Could you check a few things on this model? Use its own coordinates, in mm. Face numbers are marked on the shaded views. A direction names the side the tool comes from. Give positions to 0.01 mm unless a question says otherwise; leave off trailing zeros. Order: outer loops, then holes, each group sorted by start corner. A loop starts at its lowest first (then second) coordinate and runs counter-clockwise, first axis right, second up.
(1) If I drill on probe 1 along Z at (x, y) = (9, 15), over which ranges is the centre line in solid material (lowest first)?
(2) On a 3-axis mill with a long thin cutter (end or side, diameter ignored), from which of +Z, -Z, +X, -X, +Y, -Y can I reach the whole of each face in a straight line? I mean the marked faces 4 and 5. Say none if no direction works.
(3) Imagine slicing it at A-A, the plane x = 2. Write out the boundary of the cut face in (y, z).
(4) Will these pins go through, and if not, where does the flat tip stop? pin 1 (6 mm diameter, centred on y = 11.5, z = 2, fed in from -X); pin 2 (6 mm diameter, centred on x = 8.5, y = 12, fed in from +Z).
(5) Imagine slicing it at D-D, the plane x = 15.5. Write out the boundary of the cut face in (y, z).
(6) If we mould it in two halves opening along Y, with no side actions, what happens to the marked faces 1, 2 and 3? For each: released by +Y, released by -Y, zero draft, split by the parting line, or undercut.
(7) Imagine slicing it at B-B, the plane y = 2. Write out the boundary of the cut face in (x, z), then the cut area to 3 significant figures.
(8) Imagine slicing it at C-C, the plane y = 17.75. Write out the boundary of the cut face in (x, z).
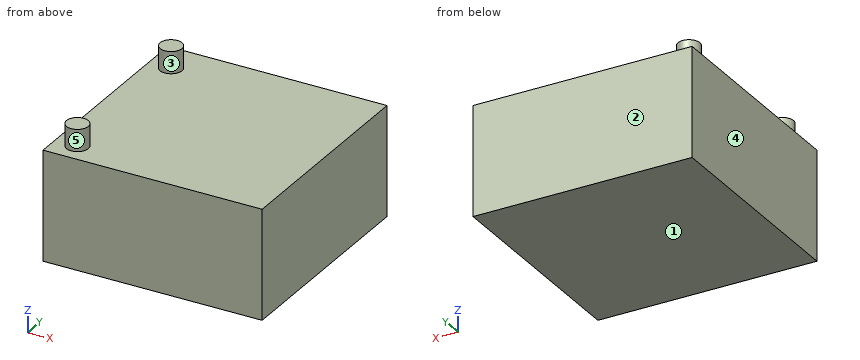
from build123d import *

# Parameters (mm, degrees)
SKETCH_1_W               = 20
SKETCH_1_H               = 20
BASEBOX_DEPTH            = 10
SKETCH_2_R               = 1
BOSSSEED_DEPTH           = 2
LINEARPATTERN_COUNT      = 2
LINEARPATTERN_PITCH      = 10
LINEARPATTERN_COUNT_DIR2 = 3
LINEARPATTERN_PITCH_DIR2 = 15


with BuildPart() as part:
    # 草图1 → BaseBox (new body)
    with BuildSketch(Plane.XY):
        with Locations((10, 10)):
            Rectangle(SKETCH_1_W, SKETCH_1_H)
    extrude(amount=BASEBOX_DEPTH)

    # 草图2 → BossSeed (add)
    with BuildSketch(Plane.XY.offset(10)):
        with Locations((2, 2)):
            Circle(SKETCH_2_R)
    bossseed = extrude(amount=BOSSSEED_DEPTH)

    # LinearPattern: BossSeed 2 × 3, 4 skipped
    with Locations(*[(-i * LINEARPATTERN_PITCH, j * LINEARPATTERN_PITCH_DIR2, 0) for i in range(LINEARPATTERN_COUNT) for j in range(LINEARPATTERN_COUNT_DIR2) if (i, j) not in ((0, 0), (0, 2), (1, 0), (1, 1), (1, 2))]):
        add(bossseed)


solid = part.part
Answer block:
1. probe 1: z = 0 to 10
2. face 4: +Z, -Z, -X, +Y, -Y
2. face 5: +Z
3. outline: (0, 0) - (20, 0) - (20, 10) - (18, 10) - (18, 12) - (16, 12) - (16, 10) - (3, 10) - (3, 12) - (1, 12) - (1, 10) - (0, 10) - close
4. pin 1: stops at x = 0
4. pin 2: stops at z = 10
5. outline: (0, 0) - (20, 0) - (20, 10) - (0, 10) - close
6. face 1: zero draft
6. face 2: released by +Y
6. face 3: undercut
7. outline: (0, 0) - (20, 0) - (20, 10) - (3, 10) - (3, 12) - (1, 12) - (1, 10) - (0, 10) - close
7. area: 204 mm2
8. outline: (0, 0) - (20, 0) - (20, 10) - (2.66, 10) - (2.66, 12) - (1.34, 12) - (1.34, 10) - (0, 10) - close
